```python
from build123d import *

# Parameters (mm, degrees)
SKETCH1_R                     = 5
BOSS_EXTRUDE1_DEPTH           = 10
BOSS_EXTRUDE1_OTHER_WAY_DEPTH = 10
BOSS_EXTRUDE1_OTHER_WAY_TAPER = 10
FILLET1_R                     = 3.85
SHELL1_T                      = -2.5


with BuildPart() as part:
    # Sketch1 → Boss-Extrude1 (new body)
    with BuildSketch(Plane(origin=(0, 0, 0), x_dir=(1, 0, 0), z_dir=(0, 1, 0))):
        with Locations(Location((0, 0, 0), (0, 0, 270))):
            Circle(SKETCH1_R)
    extrude(amount=-BOSS_EXTRUDE1_DEPTH)

    # Sketch1 → Boss-Extrude1 other way (add)
    with BuildSketch(Plane(origin=(0, 0, 0), x_dir=(1, 0, 0), z_dir=(0, 1, 0))):
        with Locations(Location((0, 0, 0), (0, 0, 270))):
            Circle(SKETCH1_R)
    extrude(amount=BOSS_EXTRUDE1_OTHER_WAY_DEPTH, taper=BOSS_EXTRUDE1_OTHER_WAY_TAPER)

    # Fillet1
    fillet1_edges = [part.edges().sort_by_distance(p)[0] for p in [
        (0, 10, -3.236730193),
    ]]
    fillet(fillet1_edges, radius=FILLET1_R)

    # Shell1
    shell1_openings = [part.faces().sort_by_distance(p)[0] for p in [
        (0, -10, 0),
    ]]
    offset(amount=SHELL1_T, openings=shell1_openings, kind=Kind.INTERSECTION)


solid = part.part
```
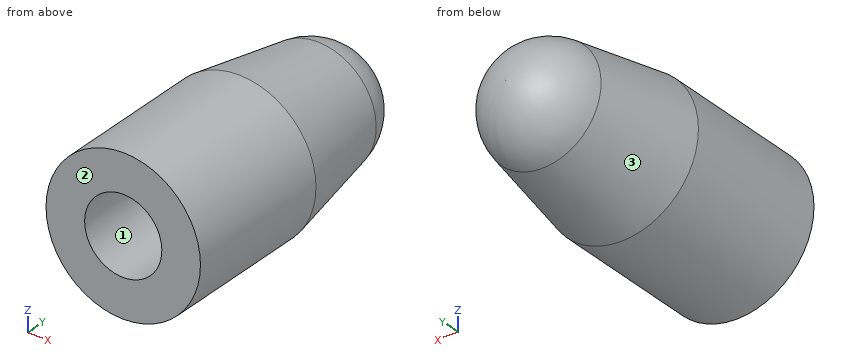
CAD build for the part. Positions are in the model's coordinates, mm. Face numbers are marked on the shaded views. Round coordinates to 2 decimals unless told otherwise and drop trailing zeros. Write each loop counter-clockwise with the first axis right and the second up, starting at its lowest first coordinate (ties: lowest second). Pieces come first, ordered by that corner, then holes.
Item 1: Band-saw the part on A-A on y = -2.5. Write the cut outline in (x, z).
Filled in:
outline: circle Ø10 at (0, 0); hole circle Ø5 at (0, 0)
Item 2: Drop flat-ended pins along their axis: pin 1 Ø3 at (y, z) = (-2.5, -2.5) entering from +X; pin 2 Ø2 at (y, z) = (-4, 2) entering from -X; pin 3 Ø1.5 at (y, z) = (-0.5, 3.5) entering from +X. Give the stop position or say it passes through.
Filled in:
pin 1: stops at x = 4.9
pin 2: stops at x = -4.9
pin 3: stops at x = 4.18
Item 3: Drill centre lines: L1, parallel to X at y = -4, z = 0; L2, parallel to X at y = 3.5, z = 0; L3, parallel to X at y = 6, z = 3. Where is each one in solid material? Low to high.
Filled in:
L1: x = -5 to -2.5, 2.5 to 5
L2: x = -4.38 to -1.84, 1.84 to 4.38
L3: x = -2.56 to 2.56
Item 4: Mould opens along X. For the marked faces 1, 2 and 3 say: released by +X, released by -X, zero draft, split by the parting line, or undercut.
Filled in:
face 1: undercut
face 2: zero draft
face 3: split by the parting line
Item 5: Band-saw the part on B-B on y = 6. Write the cut outline in (x, z).
Filled in:
outline: circle Ø7.88 at (0, 0); hole circle Ø2.81 at (0, 0)
